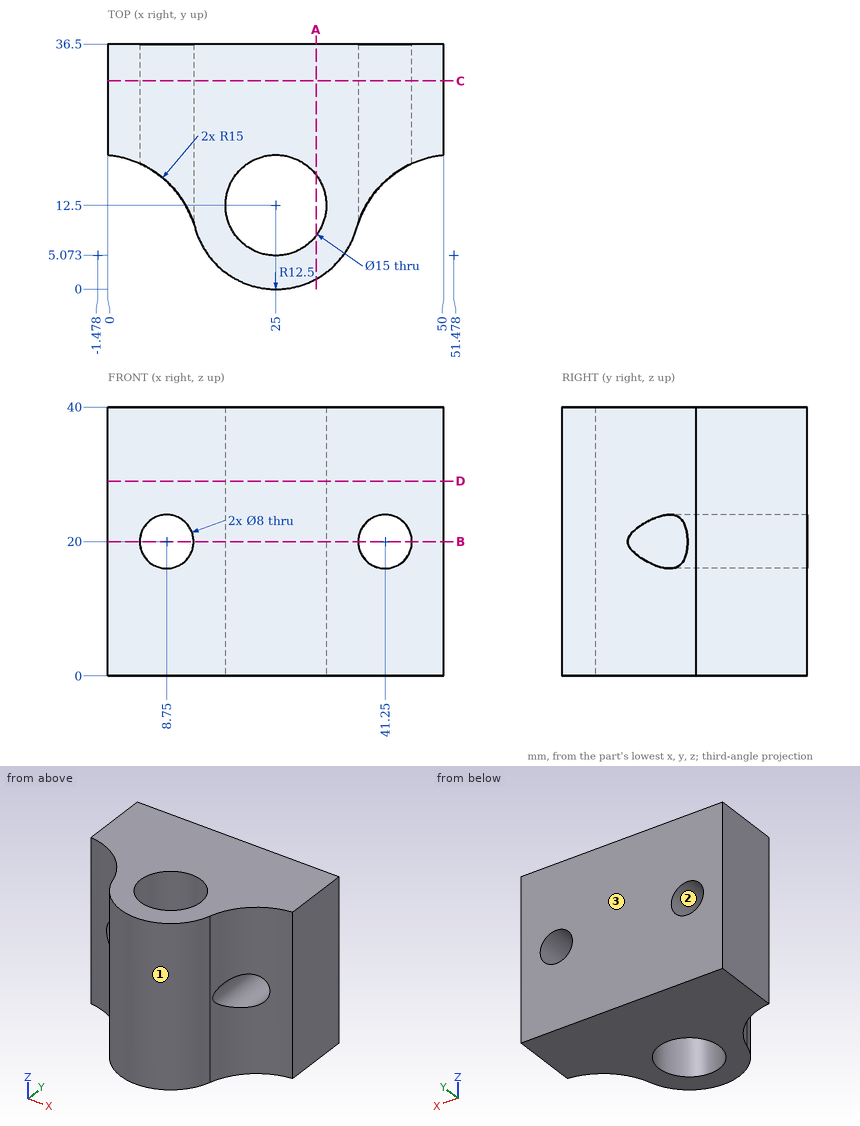
Here's the drawing with two shaded views (mm, measured from the low corner). I have some questions. Give positions to 0.01 mm unless a question says otherwise; leave off trailing zeros. Loops run counter-clockwise (first coordinate to the right, second up) from the corner with the lowest first, then second, coordinate; pieces in that order, holes last. Notation, with made-up numbers: M 7,19 L 17,19 A9 ccw 17,36 Z; hole C 88.5,-28.5 d3. An arc over 180 degrees is marked long. One line per item, written item: value.
(1) Will these pins go through, and if not, where does the flat tip stop? pin 1 (10.5 mm diameter, centred on x = 41.25, z = 20, fed in from +Y); pin 2 (4 mm diameter, centred on x = 9, y = 11, fed in from -Z); pin 3 (6 mm diameter, centred on x = 32, z = 35, fed in from -Y); pin 4 (8 mm diameter, centred on y = 11.5, z = 6, fed in from +X) (1 decimal).
Returned:
pin 1: y = 36.5
pin 2: through
pin 3: y = 0.66
pin 4: x = 40.7
(2) We'd pull the mould along X, two halves only. Please class the marked faces 1, 2 and 3: released by +X, released by -X, zero draft, split by the parting line, or undercut.
Returned:
face 1: split by the parting line
face 2: undercut
face 3: zero draft
(3) I need wall thicknesses on line 1 (Z direction, x = 9, y = 28.5); line 2 (Z direction, x = 8, y = 17); line 3 (Y direction, x = 24, z = 29). Which ranges of each line are inside material? Lowest first, please.
Returned:
line 1: 0 to 16.01, 23.99 to 40
line 2: 0 to 16.07, 23.93 to 40
line 3: 0.04 to 5.07, 19.93 to 36.5
(4) Suppose I cut it at D-D on z = 29. List the corners of the cut face in (x, y) for me, plus the area to 3 significant figures.
Returned:
outline: M 0,20 A15 cw 12.96,9.12 A12.5 ccw 37.04,9.12 A15 cw 50,20 L 50,36.5 L 0,36.5 Z; hole C 25,12.5 d15
area: 1,150 mm^2
(5) Suppose I cut it at A-A on x = 31. List the corners of the cut face in (y, z) for me, plus the area to 3 significant figures.
Returned:
outline: M 1.53,0 L 8,0 L 8,40 L 1.53,40 Z; M 17,0 L 36.5,0 L 36.5,40 L 17,40 Z
area: 1,040 mm^2
(6) Suppose I cut it at C-C on y = 31. List the corners of the cut face in (x, z) for me, plus the area to 3 significant figures.
Returned:
outline: M 0,0 L 50,0 L 50,40 L 0,40 Z; hole C 8.75,20 d8; hole C 41.25,20 d8
area: 1,900 mm^2
(7) Suppose I cut it at B-B on z = 20. List the corners of the cut face in (x, y) for me.
Returned:
outline: M 0,20 A15 cw 4.75,18.72 L 4.75,36.5 L 0,36.5 Z; M 12.75,9.82 A15 cw 12.96,9.12 A12.5 ccw 37.04,9.12 A15 cw 37.25,9.82 L 37.25,36.5 L 12.75,36.5 Z; M 45.25,18.72 A15 cw 50,20 L 50,36.5 L 45.25,36.5 Z; hole C 25,12.5 d15
